from build123d import *

# Parameters (mm, degrees)
F1_DEPTH  = 29.21
F2_W      = 15.2287210607
F2_H      = 6.9798285036
F2_W_2    = 14.8809022204
F2_H_2    = 6.6161153238
F3_DEPTH  = 12.7
F5_DEPTH  = 58.42
F7_DEPTH  = 37.677641958
F8_W      = 12.1679750076
F8_H      = 4.4820662588
F9_DEPTH  = 27.3915433795
F11_DEPTH = 14.224
F13_DEPTH = 14.224


# Not quite as in the source:
# - a feature names something its author has since deleted; it is built from what else it names


with BuildPart() as f1:
    # F0 (on Front) → F1 (new body, symmetric)
    with BuildSketch(Plane.XZ):
        Polygon((29.21, 29.21), (-29.21, 29.21), (-29.21, -11.9885886088), (-18.838820979, -11.9885886088), (-18.838820979, -28.7043564022), (-13.6548336595, -28.7043564022), (-13.6548336595, -36.2838581204), (13.73670972, -36.2838581204), (13.73670972, -28.7043564022), (18.838820979, -28.7043564022), (18.838820979, -11.9885886088), (29.21, -11.9885886088), align=None)
    extrude(amount=F1_DEPTH, both=True)

    # F2 (on face) → F3 (cut)
    with BuildSketch(Plane.XZ.offset(29.21)):
        with Locations((-14.2686051116, 10.3913402672)):
            Rectangle(F2_W, F2_H)
        with Locations((13.8336278745, 10.1568780676)):
            Rectangle(F2_W_2, F2_H_2)
    extrude(amount=-F3_DEPTH, mode=Mode.SUBTRACT)

    # F4 (on face) → F5 (cut, through all)
    with BuildSketch(Plane.XZ.offset(29.21)):
        Polygon((-11.5834288299, -13.842545168), (-11.5834288299, -24.4784541428), (-8.7825786322, -24.4784541428), (-8.7825786322, -30.5909998715), (10.1944149937, -30.5909998715), (10.1944149937, -24.4784541428), (12.9711292684, -24.4784541428), (12.9711292684, -13.8473447557), align=None)
    extrude(amount=-F5_DEPTH, mode=Mode.SUBTRACT)

    # F6 (on face) → F7 (cut, through all)
    with BuildSketch(Plane(origin=(-18.838820979, 0, 0), x_dir=(0, -1, 0), z_dir=(-1, 0, 0))):
        Polygon((20.9785699844, -12.4480193481), (-1.9933339208, -12.4480193481), (-1.9933339208, -17.8599096835), (9.0442672372, -17.8599096835), (9.0442672372, -28.7043564022), (29.3133463711, -28.7043564022), (29.3133463711, -17.8599096835), (20.9785699844, -17.8599096835), align=None)
    extrude(amount=-F7_DEPTH, mode=Mode.SUBTRACT)

    # F8 (on face) → F9 (cut, through all)
    with BuildSketch(Plane.YZ.offset(13.73670972)):
        with Locations((-19.1350400816, -30.9453895316)):
            Rectangle(F8_W, F8_H)
    extrude(amount=-F9_DEPTH, mode=Mode.SUBTRACT)

    # F10 (on face) → F11 (join)
    with BuildSketch(Plane(origin=(0, 29.21, 0), x_dir=(-1, 0, 0), z_dir=(0, 1, 0))):
        Polygon((12.8193823621, -11.6105714807), (-15.3379710391, -11.6105714807), (-15.3379710391, -26.3032335788), (-12.9711292684, -26.3032335788), (-12.9795083776, -31.884662807), (10.1667114277, -31.884662807), (10.1667114277, -26.3032335788), (12.8193823621, -26.3032335788), align=None)
    extrude(amount=-F11_DEPTH)

    # F12 (on face) → F13 (cut, through all)
    with BuildSketch(Plane(origin=(0, 29.21, 0), x_dir=(-1, 0, 0), z_dir=(0, 1, 0))):
        Polygon((6.527592428, -23.4476383775), (6.527592428, -16.5502689779), (-8.1549943425, -16.5502689779), (-8.1549943425, -23.4476383775), (-5.1418524235, -23.4476383775), (-5.1418524235, -28.0656591058), (3.516294295, -28.0656591058), (3.516294295, -23.4476383775), align=None)
    extrude(amount=-F13_DEPTH, mode=Mode.SUBTRACT)


solid = f1.part
Here's how the part is built. I have some questions about the finished solid (model axes, mm). A direction names the side the tool comes from. Round coordinates to 2 decimals unless told otherwise and drop trailing zeros. Order: outer loops, then holes, each group sorted by start corner. A loop starts at its lowest first (then second) coordinate and runs counter-clockwise, first axis right, second up. Notation, with made-up numbers: M 88,-13.75 L 139,-13.75 A26 cw 139,13.25 Z; hole C 16.25,39 d3. An arc over 180 degrees is marked long. Return JSON: item names as keys, results as strings. Group by question number.
1. Please list where these lines run through material, in increasing order: probe 1 along X at (y, z) = (-17, 11); probe 2 along Z at (x, y) = (13.5, -22.5); probe 3 along Z at (x, y) = (12, -10.5).
2. If we section it at C-C on z = -20: List the corners of the cut face in (x, y) for me (3 decimals), then the cut area to 3 significant figures.
3. If we section it at D-D on x = -16: List the corners of the cut face in (y, z) for me.
4. If we section it at B-B on y = -11.5: List the corners of the cut face in (x, z) for me, then the cut area to 3 significant figures.
5. If we mould it in two halves opening along Y, with no side actions, what happens to faces 1 (the face through (-3.516, 22, -26)), 2 (the face through (14, -16.51, 10)), 3 (the face through (-15, -3, -17.86))? For each: pulls with the +Y half, pulls with the -Y half, needs draft (parallel to the pull), parting line crosses it, or undercut.
6. On a 3-axis mill with a long thin cutter (end or side, diameter ignored), from which of +Z, -Z, +X, -X, +Y, -Y can I reach the whole of each face in a straight line? I mean faces 4 (the face through (-13.655, 0, -32)), 5 (the face through (10.194, 1, -28)), 6 (the face through (-6.528, 22, -20)), 7 (the face through (-4, -20.979, -13)), 8 (the face through (18.839, 6, -20)). Say none if no direction works.
7. I'm going to push flat-ended pins straight in: pin 1 Ø5.5 at (x, y) = (16, 5) entering from -Z; pin 2 Ø2 at (y, z) = (20.5, -20.5) entering from +X; pin 3 Ø1.5 at (x, z) = (-18.5, -27) entering from -Y; pin 4 Ø2 at (x, y) = (17.5, 8) entering from -Z. Where does each tip first touch, or does it pass through?
8. If we section it at A-A on y = -18: List the corners of the cut face in (x, z) for me.
Reply:
{
 "1": {"probe 1": "-29.21 to -21.88, -6.65 to 6.39, 21.27 to 29.21", "probe 2": "-36.28 to -33.19, -17.86 to 6.85, 13.46 to 29.21", "probe 3": "-36.28 to -28.7, -12.45 to 29.21"},
 "2": {"outline": "M -18.839,-9.044 L -11.583,-9.044 L -11.583,14.986 L -6.528,14.986 L -6.528,29.21 L -18.839,29.21 Z; M 8.155,14.986 L 12.971,14.986 L 12.971,-9.044 L 18.839,-9.044 L 18.839,29.21 L 8.155,29.21 Z", "area": "642 mm^2"},
 "3": {"outline": "M -29.21,-17.86 L -20.98,-17.86 L -20.98,-12.45 L 1.99,-12.45 L 1.99,-17.86 L -9.04,-17.86 L -9.04,-28.7 L 29.21,-28.7 L 29.21,29.21 L -29.21,29.21 L -29.21,13.88 L -16.51,13.88 L -16.51,6.9 L -29.21,6.9 Z"},
 "4": {"outline": "M -29.21,-11.99 L -18.84,-11.99 L -18.84,-12.45 L 18.84,-12.45 L 18.84,-11.99 L 29.21,-11.99 L 29.21,29.21 L -29.21,29.21 Z; M -13.65,-36.28 L 13.74,-36.28 L 13.74,-28.7 L 10.19,-28.7 L 10.19,-30.59 L -8.78,-30.59 L -8.78,-28.7 L -13.65,-28.7 Z", "area": "2,600 mm^2"},
 "5": {"face 1": "needs draft", "face 2": "pulls with the -Y half", "face 3": "undercut"},
 "6": {"face 4": "-Z, -X, +Y, -Y", "face 5": "-Y", "face 6": "+Y, -Y", "face 7": "+X, -X", "face 8": "-Z, +X, +Y, -Y"},
 "7": {"pin 1": "z = -36.28", "pin 2": "x = 18.84", "pin 3": "y = -9.04", "pin 4": "z = -28.7"},
 "8": {"outline": "M -29.21,-11.99 L -18.84,-11.99 L -18.84,-12.45 L 18.84,-12.45 L 18.84,-11.99 L 29.21,-11.99 L 29.21,29.21 L -29.21,29.21 Z; M -13.65,-36.28 L 13.74,-36.28 L 13.74,-33.19 L -13.65,-33.19 Z; hole M -21.88,6.9 L -6.65,6.9 L -6.65,13.88 L -21.88,13.88 Z; hole M 6.39,6.85 L 21.27,6.85 L 21.27,13.46 L 6.39,13.46 Z"}
}
